from build123d import *

# Parameters (mm, degrees)
F0_W      = 76.2
F0_H      = 12.7
F1_DEPTH  = 25.4
F3_DEPTH  = 50.8
F4_W      = 38.1
F4_H      = 12.7
F5_DEPTH  = 25.4
F6_W      = 12.7
F6_H      = 25.4
F7_DEPTH  = 25.4
F8_W      = 12.7
F8_H      = 50.8
F9_DEPTH  = 25.4
F10_R     = 6.35
F11_DEPTH = 25.4
F12_R     = 6.35
F13_DEPTH = 25.4


# Not quite as in the source:
# - a feature of the source that left no trace in its solid (it failed there, or was rolled back) is left out


with BuildPart() as f1:
    # F0 (on Front) → F1 (new body)
    with BuildSketch(Plane.XZ):
        with Locations((4.0105291711, 0)):
            Rectangle(F0_W, F0_H)
    extrude(amount=F1_DEPTH)

    # F0 (on Front) → F3 (join)
    with BuildSketch(Plane.XZ):
        with Locations((4.0105291711, 0)):
            Rectangle(F0_W, F0_H)
    extrude(amount=F3_DEPTH)

    # F4 (on face) → F5 (cut)
    with BuildSketch(Plane.XZ.offset(50.8)):
        with Locations((23.0605291711, 0)):
            Rectangle(F4_W, F4_H)
    extrude(amount=-F5_DEPTH, mode=Mode.SUBTRACT)

    # F6 (on face) → F7 (join)
    with BuildSketch(Plane.XY.offset(6.35)):
        with Locations((35.7605291711, -12.7)):
            Rectangle(F6_W, F6_H)
    extrude(amount=F7_DEPTH)

    # F8 (on face) → F9 (join)
    with BuildSketch(Plane.XY.offset(6.35)):
        with Locations((-27.7394708289, -25.4)):
            Rectangle(F8_W, F8_H)
    extrude(amount=F9_DEPTH)

    # F10 (on face) → F11 (cut)
    with BuildSketch(Plane.XY.offset(6.35)):
        with Locations((-8.6894708289, -37.3077057302)):
            Circle(F10_R)
    extrude(amount=-F11_DEPTH, mode=Mode.SUBTRACT)

    # F12 (on face) → F13 (cut)
    with BuildSketch(Plane.XY.offset(6.35)):
        with Locations((4.0105291711, -12.5951375812)):
            Circle(F12_R)
    extrude(amount=-F13_DEPTH, mode=Mode.SUBTRACT)


solid = f1.part
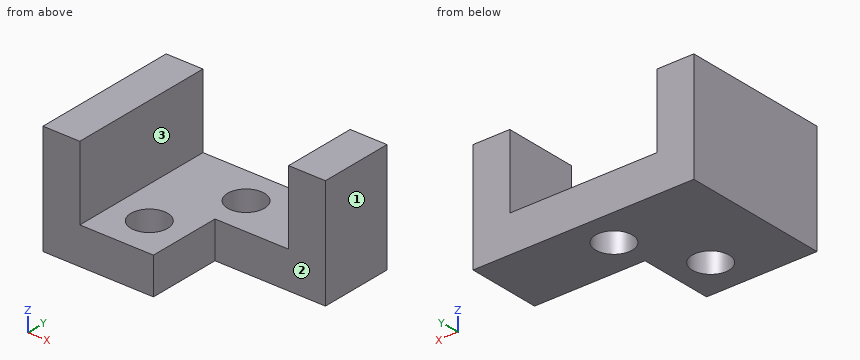
The model under review builds one solid part; all positions refer to its coordinate system, in mm. Face numbers are marked on the shaded views. A direction names the side the tool comes from. Round coordinates to 2 decimals unless told otherwise and drop trailing zeros. Order: outer loops, then holes, each group sorted by start corner. A loop starts at its lowest first (then second) coordinate and runs counter-clockwise, first axis right, second up. Notation, with made-up numbers: (56, 69.5) -> (109, 69.5) arc R23 ccw to (109, 88.5) -> close; hole circle Ø1 at (10.5, -3.75). An arc over 180 degrees is marked (long way). Use CSV: the item, a comma, the result in double quotes. Start each with the question number.
(1) Wall thickness on probe 1 along X at (y, z) = (-20, 21); probe 2 along X at (y, z) = (-49, -3); probe 3 along X at (y, z) = (-32, 21.5): over which ranges is each line inside the solid? List them lowest first. Write a range as from..to.
(2) Consider section A-A on z = 12. Write out the cut boundary in (x, y), and give its area (3 significant figures).
(3) Consider section B-B on y = -10.5. Write out the cut boundary in (x, z).
(4) Insertion check: pin 1 (1 mm diameter, centred on x = -9, y = -33, fed in from +Z); pin 2 (14.5 mm diameter, centred on x = -8.69, y = -37.31, fed in from +Z); pin 3 (3 mm diameter, centred on y = -42.5, z = 6, fed in from +X); pin 4 (11.5 mm diameter, centred on x = 24.5, z = 18, fed in from -Y). Each pin has a flat end and moves straight along its axis. Give the tip position at first contact, or say it passes through.
(5) Consider section C-C on x = -5.5. Write out the cut boundary in (y, z), and give its area (3 significant figures).
(6) Consider section D-D on y = -5. Write out the cut boundary in (x, z), and give its area (3 significant figures).
(7) Tool access review of the marked faces 1, 2 and 3: name each direction out of +Z, -Z, +X, -X, +Y, -Y from which nothing blocks a thin tool from reaching the whole face with its end or side.
Responses:
1,probe 1,"-34.09..-21.39, 29.41..42.11"
1,probe 2,"-34.09..4.01"
1,probe 3,"-34.09..-21.39"
2,outline,"(-34.09, -50.8) -> (-21.39, -50.8) -> (-21.39, 0) -> (-34.09, 0) -> close; (29.41, -25.4) -> (42.11, -25.4) -> (42.11, 0) -> (29.41, 0) -> close"
2,area,"968 mm²"
3,outline,"(-34.09, -6.35) -> (-1.98, -6.35) -> (-1.98, 6.35) -> (-21.39, 6.35) -> (-21.39, 31.75) -> (-34.09, 31.75) -> close; (10, -6.35) -> (42.11, -6.35) -> (42.11, 31.75) -> (29.41, 31.75) -> (29.41, 6.35) -> (10, 6.35) -> close"
4,pin 1,"through"
4,pin 2,"z = 6.35"
4,pin 3,"x = 4.01"
4,pin 4,"y = -25.4"
5,outline,"(-50.8, -6.35) -> (-42.8, -6.35) -> (-42.8, 6.35) -> (-50.8, 6.35) -> close; (-31.82, -6.35) -> (0, -6.35) -> (0, 6.35) -> (-31.82, 6.35) -> close"
5,area,"506 mm²"
6,outline,"(-34.09, -6.35) -> (42.11, -6.35) -> (42.11, 31.75) -> (29.41, 31.75) -> (29.41, 6.35) -> (-21.39, 6.35) -> (-21.39, 31.75) -> (-34.09, 31.75) -> close"
6,area,"1,610 mm²"
7,face 1,"+Z, -Z, +X, +Y, -Y"
7,face 2,"+Z, -Z, +X, -Y"
7,face 3,"+Z, +Y, -Y"
